Read the model definition and answer for the solid it produces. Units are mm, in the model's axes. Face numbers are marked on the shaded views. A direction names the side the tool comes from. Coordinates: 2 decimals unless noted, no trailing zeros. Loops run counter-clockwise (first coordinate to the right, second up) from the corner with the lowest first, then second, coordinate; pieces in that order, holes last. Notation, with made-up numbers: (14.25, 3.5) -> (28.25, 3.5) arc R20 ccw to (28.25, 10.5) -> close; hole circle Ø4 at (17.25, 76). An arc over 180 degrees is marked (long way). Answer as a JSON object with one key per item and string values. Group by question number.
1) Which of the six approach directions +Z, -Z, +X, -X, +Y, -Y give full straight-line access (tool end or side, diameter ignored) to the marked faces 1, 2 and 3?
2) Section B-B, the plane x = 0 is taken. Give the vertices of the cut face in (y, z), plus the area to 3 significant figures.
3) Flat-ended cylindrical pins translate along their axes: P1, Ø1.7, axis at x = -0.5, y = 0, coming from the -Z side; P2, Ø1, axis at x = -1.5, y = -1.5, coming from the +Z side; P3, Ø0.8, axis at x = -1.5, z = 0.5, coming from the +Y side; P4, Ø1.5, axis at x = -0.5, z = 3.5, coming from the +Y side. Find the tip coordinate at first contact, or state that the pin passes through.
4) Consider probe 1 along Y at (x, z) = (0, 2.65); probe 2 along X at (y, z) = (-0.9, 4.5). Determine where each line is inside the solid, lowest interval first. Write a range as [from, to].
5) Section C-C, the plane z = 9.5 is taken. Give the vertices of the cut face in (x, y), plus the area to 3 significant figures.
6) Section A-A, the plane y = 0 is taken. Give the vertices of the cut face in (x, z), plus the area to 3 significant figures.
7) Determine the mould class of the marked faces 4, 5 and 6 for opening direction X: released by +X, released by -X, zero draft, split by the parting line, or undercut.
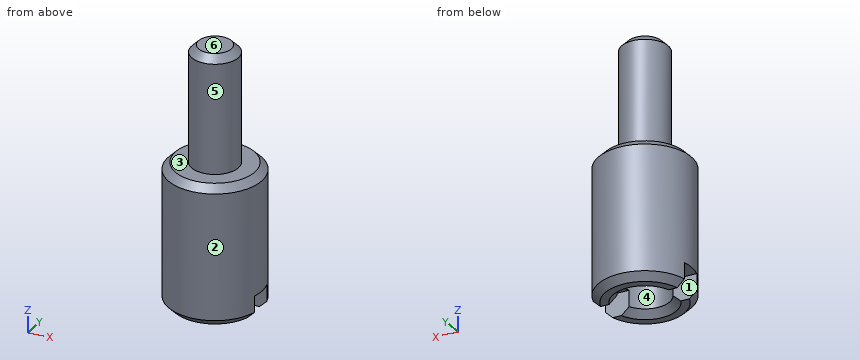
Autodesk Inventor part; units mm, degrees
ref_plane "YZ Plane" through (0, 0, 0) normal (1, 0, 0) x (0, 1, 0)
ref_plane "XZ Plane" through (0, 0, 0) normal (0, 1, 0) x (-1, 0, 0)
ref_plane "XY Plane" through (0, 0, 0) normal (0, 0, 1) x (1, 0, 0)
sketch "Sketch1" plane through (0, 0, 0) normal (0, 1, 0) x (-1, 0, 0)
  line L0 (0, 0) -> (-2, 0)
  line L1 (-2, 0) -> (-2, 6)
  line L2 (-2, 6) -> (-1, 6)
  line L3 (-1, 6) -> (-1, 11)
  line L4 (-1, 11) -> (0, 11)
  line L5 (0, 11) -> (0, 0)
  dimension "d1" = 5
  dimension "d2" = 6
  dimension "d3" = 2
  dimension "d4" = 4
revolve "Revolution1" add sketch "Sketch1" angle 360 about axis through (0, 0, 11) along (0, 0, -1)
sketch "Sketch2" plane through (0, 0, 0) normal (0, 0, -1) x (-1, 0, 0)
  line L0 (-2, -0.5) -> (2, -0.5)
  line L1 (2, -0.5) -> (2, 0.5)
  line L2 (2, 0.5) -> (-2, 0.5)
  line L3 (-2, 0.5) -> (-2, -0.5)
  line L4 (-2, -0.5) -> (2, 0.5) construction
  line L5 (2, -0.5) -> (-2, 0.5) construction
  circle A0 centre (0, 0) radius 2
  dimension "d6" = 1
extrude "Extrusion1" cut sketch "Sketch2" against normal blind 1 contours L3 A0 L0 | A0 L2 L0 | L3 L2 A0 | A0 L1 L0 | A0 L2 L1
hole "Hole1" at (0, 0, 0) direction (0, 0, 1) diameter 2.1129 depth 5
thread "Thread1"
chamfer "Chamfer1" distance 0.3 angle 45 7 edges at (-2, 0, 6) (0, 2, 0) (0, -2, 0) (0, -1.0564, 0) (-0.5421, 0.9067, 0) (0.5421, 0.9067, 0) (-1, 0, 11)
properties part number "BRU-2006S" material "Stainless Steel AISI 304"
Determined:
{
 "1": {"face 1": "-Z, +X, -X", "face 2": "+Z, -Z", "face 3": "+Z"},
 "2": {"outline": "(-2, 0.3) -> (-1.7, 0) -> (-1.36, 0) -> (-1.06, 0.3) -> (-1.06, 5) -> (1.06, 5) -> (1.06, 0.3) -> (1.36, 0) -> (1.7, 0) -> (2, 0.3) -> (2, 5.7) -> (1.7, 6) -> (1, 6) -> (1, 10.7) -> (0.7, 11) -> (-0.7, 11) -> (-1, 10.7) -> (-1, 6) -> (-1.7, 6) -> (-2, 5.7) -> close", "area": "23.1 mm²"},
 "3": {"P1": "z = 0.07", "P2": "z = 6", "P3": "y = 1.67", "P4": "y = 2"},
 "4": {"probe 1": "[-2, -1.06], [1.06, 2]", "probe 2": "[-1.79, -0.55], [0.55, 1.79]"},
 "5": {"outline": "circle Ø2 at (0, 0)", "area": "3.14 mm²"},
 "6": {"outline": "(-2, 1) -> (-1.06, 1) -> (-1.06, 5) -> (1.06, 5) -> (1.06, 1) -> (2, 1) -> (2, 5.7) -> (1.7, 6) -> (1, 6) -> (1, 10.7) -> (0.7, 11) -> (-0.7, 11) -> (-1, 10.7) -> (-1, 6) -> (-1.7, 6) -> (-2, 5.7) -> close", "area": "21.4 mm²"},
 "7": {"face 4": "undercut", "face 5": "split by the parting line", "face 6": "zero draft"}
}
